For this review, take the finished solid that the model builds, in its own axes (mm). Face numbers are marked on the shaded views. A direction names the side the tool comes from. Coordinates: 2 decimals unless noted, no trailing zeros. Loops run counter-clockwise (first coordinate to the right, second up) from the corner with the lowest first, then second, coordinate; pieces in that order, holes last. Notation, with made-up numbers: (28, 26) -> (48, 26) arc R24 cw to (48, 46) -> close; hole circle Ø5 at (-39.75, 84). An arc over 180 degrees is marked (long way). Answer in a Markdown table with one row per item.
from build123d import *

# Parameters (mm, degrees)
SKETCH1_W           = 30
SKETCH1_H           = 75
BOSS_EXTRUDE1_DEPTH = 12
CUT_EXTRUDE1_DEPTH  = 12
LPATTERN1_COUNT     = 3
LPATTERN1_PITCH     = 20
BOUNDARY1_START     = -45
BOUNDARY1_DEPTH     = 5
LPATTERN2_COUNT     = 9
LPATTERN2_PITCH     = 5


# Read off the part's stored shape, not the designer's step: Boundary1
with BuildPart() as part:
    # Sketch1 → Boss-Extrude1 (new body)
    with BuildSketch(Plane(origin=(0, 0, 0), x_dir=(1, 0, 0), z_dir=(0, 1, 0))):
        with Locations((15, 37.5)):
            Rectangle(SKETCH1_W, SKETCH1_H)
    extrude(amount=BOSS_EXTRUDE1_DEPTH)

    # Sketch3 → Cut-Extrude1 (cut)
    with BuildSketch(Plane(origin=(0, 0, 0), x_dir=(1, 0, 0), z_dir=(0, 1, 0))):
        Polygon((0, 5), (22.5, 12.5), (0, 20), align=None)
    cut_extrude1 = extrude(amount=CUT_EXTRUDE1_DEPTH, mode=Mode.SUBTRACT)

    # LPattern1: Cut-Extrude1 ×3
    with Locations(*[(0, 0, -i * LPATTERN1_PITCH) for i in range(1, LPATTERN1_COUNT)]):
        add(cut_extrude1, mode=Mode.SUBTRACT)

    # Boundary1 outline → Boundary1 (add)
    with BuildSketch(Plane.XY.offset(BOUNDARY1_START)):
        Polygon((30, 0), (25, 0), (30, -2), align=None)
    boundary1 = extrude(amount=BOUNDARY1_DEPTH)

    # LPattern2: Boundary1 ×9
    with Locations(*[(0, 0, i * LPATTERN2_PITCH) for i in range(1, LPATTERN2_COUNT)]):
        add(boundary1)


solid = part.part
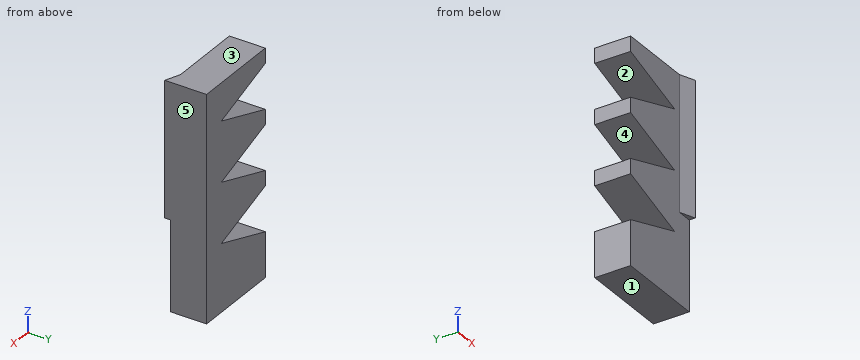
Item 1: The part is to be moulded in two halves that separate along Z. For the marked faces 3, 4 and 5, say which applies: +Z half, -Z half, draft (parallel to the pull), parting line (faces both ways), or undercut.
Worked answers:
| item | result |
|---|---|
| face 3 | +Z half |
| face 4 | undercut |
| face 5 | draft |
Item 2: Take a section at C-C, the plane y = 2. State the section outline as (x, z) points.
Worked answers:
| item | result |
|---|---|
| outline | (0, -75) -> (30, -75) -> (30, 0) -> (0, 0) -> (0, -5) -> (22.5, -12.5) -> (0, -20) -> (0, -25) -> (22.5, -32.5) -> (0, -40) -> (0, -45) -> (22.5, -52.5) -> (0, -60) -> close |
Item 3: For L1, parallel to Z at x = 21.5, y = 11.5; L2, parallel to Z at x = 8.5, y = 4.25; L3, parallel to Y at x = 19.5, z = -48.5, list the stretches that pass through material, from the lowest coordinate up.
Worked answers:
| item | result |
|---|---|
| L1 | -75 to -52.83, -52.17 to -32.83, -32.17 to -12.83, -12.17 to 0 |
| L2 | -75 to -57.17, -47.83 to -37.17, -27.83 to -17.17, -7.83 to 0 |
| L3 | 0 to 12 |
Item 4: Insertion check: pin 1 (1.5 mm diameter, centred on y = 6, z = -39.5, fed in from -X); pin 2 (15 mm diameter, centred on x = 20.5, z = -30.5, fed in from -Y); pin 3 (4 mm diameter, centred on x = 17, z = -18.5, fed in from -Y). Each pin has a flat end and moves straight along its axis. Give the tip position at first contact, or say it passes through.
Worked answers:
| item | result |
|---|---|
| pin 1 | x = 0 |
| pin 2 | y = -1.2 |
| pin 3 | y = 0 |
Item 5: Take a section at B-B, the plane z = -42. State the section outline as (x, y) points, and give its area (3 significant figures).
Worked answers:
| item | result |
|---|---|
| outline | (0, 0) -> (25, 0) -> (30, -2) -> (30, 12) -> (0, 12) -> close |
| area | 365 mm² |
Item 6: Take a section at D-D, the plane x = 16.5. State the section outline as (y, z) points, and give its area (3 significant figures).
Worked answers:
| item | result |
|---|---|
| outline | (0, -75) -> (12, -75) -> (12, -54.5) -> (0, -54.5) -> close; (0, -50.5) -> (12, -50.5) -> (12, -34.5) -> (0, -34.5) -> close; (0, -30.5) -> (12, -30.5) -> (12, -14.5) -> (0, -14.5) -> close; (0, -10.5) -> (12, -10.5) -> (12, 0) -> (0, 0) -> close |
| area | 756 mm² |
Item 7: For the marked faces 1 and 2, list the 3-axis set-ups (+Z, -Z, +X, -X, +Y, -Y) from which the entire face can be reached by the end or side of a thin tool; tool diameter is ignored.
Worked answers:
| item | result |
|---|---|
| face 1 | -Z, +X, -X, +Y, -Y |
| face 2 | -X, +Y, -Y |
Item 8: Take a section at A-A, the plane x = 12. State the section outline as (y, z) points.
Worked answers:
| item | result |
|---|---|
| outline | (0, -75) -> (12, -75) -> (12, -56) -> (0, -56) -> close; (0, -49) -> (12, -49) -> (12, -36) -> (0, -36) -> close; (0, -29) -> (12, -29) -> (12, -16) -> (0, -16) -> close; (0, -9) -> (12, -9) -> (12, 0) -> (0, 0) -> close |
